Geometry: final body of the model. Coordinates: model frame, mm. A direction names the side the tool comes from. Give positions to 0.01 mm unless a question says otherwise; leave off trailing zeros. Write each loop counter-clockwise with the first axis right and the second up, starting at its lowest first coordinate (ties: lowest second). Pieces come first, ordered by that corner, then holes.
```python
from build123d import *

# Parameters (mm, degrees)
SKETCH1_W                = 9
SKETCH1_H                = 1
BOSS_EXTRUDE1_DEPTH      = 4.5
BOSS_EXTRUDE2_DEPTH      = 2.1
BOSS_EXTRUDE2_DEPTH_BACK = 1
FILLET1_R                = 0.255
SKETCH3_W                = 1
SKETCH3_H                = 3.438773138
SKETCH3_W_2              = 2.5
SKETCH3_H_2              = 3.613088827
SKETCH3_W_3              = 2.495866097
SKETCH3_H_3              = 3.882485801
CUT_EXTRUDE1_DEPTH       = 9
CHAMFER1_SIZE            = 0.75
CHAMFER1_SIZE2           = 2.378696102
SKETCH4_W                = 1
SKETCH4_H                = 2.4
BOSS_EXTRUDE3_DEPTH      = 1.7
SKETCH5_W                = 0.75
SKETCH5_H                = 0.75
CUT_EXTRUDE2_DEPTH       = 10.85
CHAMFER2_SIZE            = 0.75
SKETCH6_W                = 3.885576696
SKETCH6_H                = 1.699016426
SKETCH6_W_2              = 2.747974394
SKETCH6_H_2              = 0.842121185
CUT_EXTRUDE3_DEPTH       = 21.7
FILLET2_R                = 0.1


with BuildPart() as part:
    # Sketch1 → Boss-Extrude1 (new, symmetric)
    with BuildSketch(Plane.XY):
        Rectangle(SKETCH1_W, SKETCH1_H)
    extrude(amount=BOSS_EXTRUDE1_DEPTH, both=True)

    # Sketch2 → Boss-Extrude2 (add, two sides: drawn at the far end of the back side and taken through both)
    with BuildSketch(Plane(origin=(0, 0.5, 0), x_dir=(1, 0, 0), z_dir=(0, 1, 0)).offset(-BOSS_EXTRUDE2_DEPTH_BACK)):
        with BuildLine():
            Line((-4.5, -4.5), (-4.5, -5))
            ThreePointArc((-4.5, -5), (0, -5.438805544), (4.5, -5))
            Line((4.5, -5), (4.5, -4.5))
            Line((4.5, -4.5), (-4.5, -4.5))
        make_face()
    extrude(amount=BOSS_EXTRUDE2_DEPTH + BOSS_EXTRUDE2_DEPTH_BACK)

    # Fillet1
    fillet1_edges = [part.edges().sort_by_distance(p)[0] for p in [
        (0, 2.6, 4.5),
        (4.5, 2.6, 4.75),
        (0, 2.6, 5.438805544),
        (-4.5, 2.6, 4.75),
        (4.5, 1.55, 4.5),
        (-4.5, 1.55, 4.5),
        (4.5, 1.05, 5),
        (-4.5, 1.05, 5),
    ]]
    fillet(fillet1_edges, radius=FILLET1_R)

    # Sketch3 → Cut-Extrude1 (cut)
    with BuildSketch(Plane(origin=(0, 0.5, 0), x_dir=(1, 0, 0), z_dir=(0, 1, 0))):
        with Locations((3, 3.819386569)):
            Rectangle(SKETCH3_W, SKETCH3_H)
        with Locations((-1.25, 3.906544413)):
            Rectangle(SKETCH3_W_2, SKETCH3_H_2)
        with Locations((-4.747933049, 4.041242901)):
            Rectangle(SKETCH3_W_3, SKETCH3_H_3)
    extrude(amount=-CUT_EXTRUDE1_DEPTH, mode=Mode.SUBTRACT)

    # Chamfer1
    chamfer1_edges = [part.edges().sort_by_distance(p)[0] for p in [
        (1.25, 0.5, -4.5),
    ]]
    chamfer1_side = [part.faces().sort_by_distance(p)[0] for p in [
        (1.25, 0, -4.5),
    ]]
    chamfer(chamfer1_edges, length=CHAMFER1_SIZE, length2=CHAMFER1_SIZE2, reference=chamfer1_side[0])

    # Sketch4 → Boss-Extrude3 (add)
    with BuildSketch(Plane(origin=(0, 0.5, 0), x_dir=(1, 0, 0), z_dir=(0, 1, 0))):
        with Locations((4, 3.3)):
            Rectangle(SKETCH4_W, SKETCH4_H)
        with Locations((-3, 3.3)):
            Rectangle(SKETCH4_W, SKETCH4_H)
    extrude(amount=BOSS_EXTRUDE3_DEPTH)

    # Sketch5 → Cut-Extrude2 (cut, symmetric)
    with BuildSketch(Plane.ZY.offset(-3.5)):
        with Locations((-2.475, 0.875)):
            Rectangle(SKETCH5_W, SKETCH5_H)
    extrude(amount=CUT_EXTRUDE2_DEPTH, both=True, mode=Mode.SUBTRACT)

    # Chamfer2
    chamfer2_edges = [part.edges().sort_by_distance(p)[0] for p in [
        (4, 2.2, -2.1),
        (-3, 2.2, -2.1),
    ]]
    chamfer(chamfer2_edges, length=CHAMFER2_SIZE)

    # Sketch6 → Cut-Extrude3 (cut)
    with BuildSketch(Plane(origin=(0, 2.2, 0), x_dir=(1, 0, 0), z_dir=(0, 1, 0))):
        with Locations((-3.730449109, 4.599508213)):
            Rectangle(SKETCH6_W, SKETCH6_H)
        with Locations((4.565183266, 4.171060592)):
            Rectangle(SKETCH6_W_2, SKETCH6_H_2)
    extrude(amount=-CUT_EXTRUDE3_DEPTH, mode=Mode.SUBTRACT)

    # Fillet2
    fillet2_edges = [part.edges().sort_by_distance(p)[0] for p in [
        (-3.5, -0.5, -2.925),
        (-4.5, 0, -2.1),
        (-4, -0.5, -2.1),
        (-2.5, -0.5, -2.925),
        (-3, -0.5, -3.75),
        (4, -0.5, -3.75),
        (4.5, -0.5, 0.519670946),
        (0, -0.5, 5.438805544),
        (-4.5, -0.5, 1.344670946),
        (-4.441222256, -0.5, 4.952197123),
        (4.441222256, -0.5, 4.952197123),
        (-4.5, 0.5, 1.3275),
        (3, -0.5, -2.1),
        (4.5, 0.5, 0.9525),
        (2.5, -0.5, -3.3),
        (3.5, -0.5, -2.925),
        (1.25, -0.5, -4.5),
        (0, -0.5, -3.3),
        (-1.25, -0.5, -2.1),
    ]]
    fillet(fillet2_edges, radius=FILLET2_R)


solid = part.part
```
Item 1: Section A-A, the plane y = 2. Return the cut outline in (x, z) (3 decimals).
Found:
outline: (-4.5, 4.755) arc R0.255 ccw to (-4.245, 4.5) - (4.245, 4.5) arc R0.255 ccw to (4.5, 4.755) - (4.5, 4.789) arc R0.255 ccw to (4.292, 5.04) arc R23.293 ccw to (-4.292, 5.04) arc R0.255 ccw to (-4.5, 4.789) - close; (-3.5, -3.75) - (-2.5, -3.75) - (-2.5, -2.65) - (-3.5, -2.65) - close; (3.5, -3.75) - (4.5, -3.75) - (4.5, -2.65) - (3.5, -2.65) - close
Item 2: Section B-B, the plane z = -2.25. Return the cut outline in (x, y).
Found:
outline: (-3.5, -0.4) arc R0.1 ccw to (-3.4, -0.5) - (-2.6, -0.5) arc R0.1 ccw to (-2.5, -0.4) - (-2.5, 0.5) - (-3.5, 0.5) - close; (-3.5, 1.25) - (-2.5, 1.25) - (-2.5, 1.6) - (-3.5, 1.6) - close; (0, -0.4) arc R0.1 ccw to (0.1, -0.5) - (2.4, -0.5) arc R0.1 ccw to (2.5, -0.4) - (2.5, 0.46) - (0, 0.46) - close; (3.5, -0.4) arc R0.1 ccw to (3.6, -0.5) - (4.4, -0.5) arc R0.1 ccw to (4.5, -0.4) - (4.5, 0.4) arc R0.1 ccw to (4.4, 0.5) - (3.5, 0.5) - close; (3.5, 1.25) - (4.5, 1.25) - (4.5, 1.6) - (3.5, 1.6) - close
Item 3: Reachability of faces 4 (the face through (3.5, 0.9, -3.1)), 5 (the face through (1.23, 0.13, -3.29)), 6 (the face through (4, 2.2, -3)) from +Z, -Z, +X, -X, +Y, -Y: full face, straight path, thin tool, end or side. Return the list, or none.
Found:
face 4: -Z, +Y, -Y
face 5: -Z, +Y
face 6: -Z, +X, -X, +Y
Item 4: Pull-direction query (Z, two-part tool) for faces 1 (the face through (0, -0.5, 1)), 2 (the face through (0, 0.5, 1)), 3 (the face through (-0.06, 0.95, 5.44)); classes: +Z half, -Z half, draft (parallel to the pull), parting line (faces both ways), or undercut.
Found:
face 1: draft
face 2: undercut
face 3: +Z half
Item 5: Line query: L1, parallel to Y at x = 4, z = -3; L2, parallel to Y at x = -1.75, z = -1.25; L3, parallel to Z at x = -2.75, y = 1.85. Output: solid intervals per line, ascending.
Found:
L1: y = -0.5 to 2.2
L2: y = -0.5 to 0.5
L3: z = -3.75 to -2.5, 4.5 to 5.28
Item 6: Pin query (flat end, axial travel): pin 1 Ø1.1 at (x, y) = (4, 1.5) entering from -Z; pin 2 Ø0.5 at (y, z) = (0.5, -2.5) entering from -X; pin 3 Ø0.5 at (x, y) = (-3, 0.5) entering from -Z. Return the tip coordinate at first contact, or that it passes through.
Found:
pin 1: stops at z = -3.75
pin 2: stops at x = -3.5
pin 3: stops at z = -3.75
Item 7: Section C-C, the plane z = 2.75. Return the cut outline in (x, y), plus the area to 3 significant figures.
Found:
outline: (-4.5, -0.4) arc R0.1 ccw to (-4.4, -0.5) - (4.4, -0.5) arc R0.1 ccw to (4.5, -0.4) - (4.5, 0.4) arc R0.1 ccw to (4.4, 0.5) - (-4.4, 0.5) arc R0.1 ccw to (-4.5, 0.4) - close
area: 8.99 mm2
Item 8: Section D-D, the plane y = 0.9. Return the cut outline in (x, z) (3 decimals), plus the area to 3 significant figures.
Found:
outline: (-4.5, 4.755) arc R0.255 ccw to (-4.245, 4.5) - (4.245, 4.5) arc R0.255 ccw to (4.5, 4.755) - (4.5, 4.789) arc R0.255 ccw to (4.292, 5.04) arc R23.293 ccw to (-4.292, 5.04) arc R0.255 ccw to (-4.5, 4.789) - close; (-3.5, -3.75) - (-2.5, -3.75) - (-2.5, -2.85) - (-3.5, -2.85) - close; (3.5, -3.75) - (4.5, -3.75) - (4.5, -2.85) - (3.5, -2.85) - close
area: 8.89 mm2
